Can you work these out from the model? Positions are in its coordinate system, mm. Face numbers are marked on the shaded views. A direction names the side the tool comes from. Round coordinates to 2 decimals unless told otherwise and drop trailing zeros. Loops run counter-clockwise (first coordinate to the right, second up) from the corner with the lowest first, then second, coordinate; pieces in that order, holes last. Notation, with made-up numbers: M 74.25,24.25 L 93.25,24.25 A12 cw 93.25,37.25 Z; hole C 63.25,2 d10. An arc over 180 degrees is marked long. Answer as CSV lines item,"result".
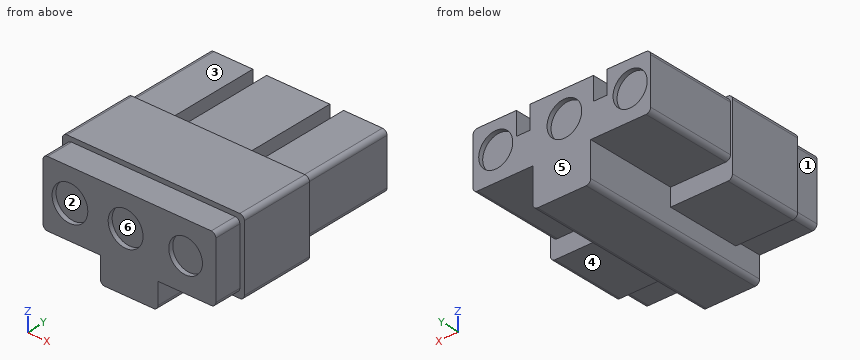
from build123d import *

# Parameters (mm, degrees)
SKETCH_1_W          = 39.8
SKETCH_1_H          = 16.4
EXTRUDE_1_DEPTH     = 16.3
SKETCH_2_W          = 37.8
SKETCH_2_H          = 14.4
EXTRUDE_2_DEPTH     = 6
SKETCH_3_W          = 38.834721862
SKETCH_3_H          = 12.135850582
EXTRUDE_3_DEPTH     = 20
SKETCH_4_W          = 12.623118615
SKETCH_4_H          = 42.3
EXTRUDE_4_DEPTH     = 8.5
SKETCH_5_W          = 3
SKETCH_5_H          = 20
CUT_EXTRUDE_2_DEPTH = 5
SKETCH_6_R          = 3.734555691
SKETCH_6_R_2        = 3.793211722
SKETCH_6_R_3        = 3.72240449
CUT_EXTRUDE_3_DEPTH = 1
SKETCH_7_R          = 3.906226906
SKETCH_7_R_2        = 3.81532866
SKETCH_7_R_3        = 3.686295828
CUT_EXTRUDE_4_DEPTH = 1
FILLET_1_R          = 1


with BuildPart() as part:
    # ｽｹｯﾁ1 → ﾎﾞｽ - 押し出し1 (new body)
    with BuildSketch(Plane(origin=(0, 0, 0), x_dir=(1, 0, 0), z_dir=(0, 1, 0))):
        with Locations((19.9, 8.2)):
            Rectangle(SKETCH_1_W, SKETCH_1_H)
    extrude(amount=EXTRUDE_1_DEPTH)

    # ｽｹｯﾁ2 → ﾎﾞｽ - 押し出し2 (add)
    with BuildSketch(Plane.XZ):
        with Locations((19.9, -8.2)):
            Rectangle(SKETCH_2_W, SKETCH_2_H)
    extrude(amount=EXTRUDE_2_DEPTH)

    # ｽｹｯﾁ3 → ﾎﾞｽ - 押し出し3 (add)
    with BuildSketch(Plane(origin=(0, 16.3, 0), x_dir=(1, 0, 0), z_dir=(0, 1, 0))):
        with Locations((19.862075467, 6.474433745)):
            Rectangle(SKETCH_3_W, SKETCH_3_H)
    extrude(amount=EXTRUDE_3_DEPTH)

    # ｽｹｯﾁ4 → ﾎﾞｽ - 押し出し4 (add)
    with BuildSketch(Plane(origin=(0, 0, -12.542359036), x_dir=(-1, 0, 0), z_dir=(0, 0, -1))):
        with Locations((-19.847838353, 15.15)):
            Rectangle(SKETCH_4_W, SKETCH_4_H)
    extrude(amount=EXTRUDE_4_DEPTH)

    # ｽｹｯﾁ5 → ｶｯﾄ - 押し出し2 (cut)
    with BuildSketch(Plane.XY.offset(-0.406508454)):
        with Locations((11.444714536, 26.3)):
            Rectangle(SKETCH_5_W, SKETCH_5_H)
        with Locations((28.279436398, 26.3)):
            Rectangle(SKETCH_5_W, SKETCH_5_H)
    extrude(amount=-CUT_EXTRUDE_2_DEPTH, mode=Mode.SUBTRACT)

    # ｽｹｯﾁ6 → ｶｯﾄ - 押し出し3 (cut)
    with BuildSketch(Plane(origin=(0, 36.3, 0), x_dir=(1, 0, 0), z_dir=(0, 1, 0))):
        with Locations(Location((4.919809438, 6.178820482, 0), (0, 0, 270))):
            Circle(SKETCH_6_R)
        with Locations(Location((19.293207471, 6.178820482, 0), (0, 0, 270))):
            Circle(SKETCH_6_R_2)
        with Locations(Location((34.311322566, 6.178820482, 0), (0, 0, 270))):
            Circle(SKETCH_6_R_3)
    extrude(amount=-CUT_EXTRUDE_3_DEPTH, mode=Mode.SUBTRACT)

    # ｽｹｯﾁ7 → ｶｯﾄ - 押し出し4 (cut)
    with BuildSketch(Plane.XZ.offset(6)):
        with Locations(Location((6.891885157, -8.075047135, 0), (0, 0, 270))):
            Circle(SKETCH_7_R)
        with Locations(Location((19.065660272, -8.075047135, 0), (0, 0, 270))):
            Circle(SKETCH_7_R_2)
        with Locations(Location((32.187548714, -8.075047135, 0), (0, 0, 270))):
            Circle(SKETCH_7_R_3)
    extrude(amount=-CUT_EXTRUDE_4_DEPTH, mode=Mode.SUBTRACT)

    # ﾌｨﾚｯﾄ1
    fillet_1_edges = [part.edges().sort_by_distance(p)[0] for p in [
        (38.8, -3, -1),
        (1, -3, -1),
        (1, -3, -15.4),
        (38.8, -3, -15.4),
        (0.444714536, 26.3, -12.542359036),
        (0.444714536, 26.3, -0.406508454),
        (39.279436398, 26.3, -0.406508454),
        (39.279436398, 26.3, -12.542359036),
        (26.15939766, 15.15, -21.042359036),
        (13.536279045, 15.15, -21.042359036),
        (0, 8.15, -16.4),
        (39.8, 8.15, -16.4),
        (39.8, 8.15, 0),
        (0, 8.15, 0),
    ]]
    fillet(fillet_1_edges, radius=FILLET_1_R)


solid = part.part
Item 1: If I drill on line 1 along X through (y, z) = (32.5, -4); line 2 along Z through (x, y) = (27, 27); line 3 along Z through (x, y) = (23, 30), over which ranges is the centre line in solid material (lowest first)? Write a range as from..to.
Output:
line 1,"x = 0.44..9.94, 12.94..26.78, 29.78..39.28"
line 2,"z = -12.54..-5.41"
line 3,"z = -21.04..-0.41"
Item 2: If we section it at C-C on z = -17.25: Write out the boundary of the cut face in (x, y).
Output:
outline,"M 13.54,-6 L 26.16,-6 L 26.16,36.3 L 13.54,36.3 Z"
Item 3: If we section it at D-D on y = 5.5: Write out the boundary of the cut face in (x, z), then the cut area to 3 significant figures.
Output:
outline,"M 0,-15.4 A1 ccw 1,-16.4 L 13.54,-16.4 L 13.54,-20.04 A1 ccw 14.54,-21.04 L 25.16,-21.04 A1 ccw 26.16,-20.04 L 26.16,-16.4 L 38.8,-16.4 A1 ccw 39.8,-15.4 L 39.8,-1 A1 ccw 38.8,0 L 1,0 A1 ccw 0,-1 Z"
area,"710 mm2"
Item 4: Will these pins go through, and if not, where does the flat tip stop? pin 1 (8 mm diameter, centred on y = 25, z = -10, fed in from +X); pin 2 (4 mm diameter, centred on x = 8, y = 5.5, fed in from -Z); pin 3 (4 mm diameter, centred on x = 6, z = -7.5, fed in from -Y); pin 4 (8.5 mm diameter, centred on x = 32.19, z = -8.08, fed in from +Y).
Output:
pin 1,"stops at x = 39.28"
pin 2,"stops at z = -16.4"
pin 3,"stops at y = -5"
pin 4,"stops at y = 36.3"
Item 5: On a 3-axis mill with a long thin cutter (end or side, diameter ignored), from which of +Z, -Z, +X, -X, +Y, -Y can I reach the whole of each face in a straight line? I mean the marked faces 1, 2 and 3. Say none if no direction works.
Output:
face 1,"+Z, -Z, -X, -Y"
face 2,"-Y"
face 3,"+Z, +X, -X, +Y"
Item 6: If we section it at A-A on y = -0.5: Write out the boundary of the cut face in (x, z).
Output:
outline,"M 1,-14.4 A1 ccw 2,-15.4 L 13.54,-15.4 L 13.54,-20.04 A1 ccw 14.54,-21.04 L 25.16,-21.04 A1 ccw 26.16,-20.04 L 26.16,-15.4 L 37.8,-15.4 A1 ccw 38.8,-14.4 L 38.8,-2 A1 ccw 37.8,-1 L 2,-1 A1 ccw 1,-2 Z"
Item 7: We'd pull the mould along Z, two halves only. Please class the marked faces 4, 5 and 6: released by +Z, released by -Z, zero draft, split by the parting line, or undercut.
Output:
face 4,"released by -Z"
face 5,"zero draft"
face 6,"undercut"
Item 8: If we section it at B-B on x = 36.5: Write out the boundary of the cut face in (y, z).
Output:
outline,"M -6,-15.4 L 0,-15.4 L 0,-16.4 L 16.3,-16.4 L 16.3,-12.54 L 36.3,-12.54 L 36.3,-9.19 L 35.3,-9.19 L 35.3,-3.17 L 36.3,-3.17 L 36.3,-0.41 L 16.3,-0.41 L 16.3,0 L 0,0 L 0,-1 L -6,-1 Z"
